```python
from build123d import *

# Parameters (mm, degrees)
BOSS_EXTRUDE1_DEPTH = 152.146
SKETCH2_W           = 2.509536254
SKETCH2_H           = 5.091968042
SKETCH2_W_2         = 2.457399938
BOSS_EXTRUDE2_DEPTH = 2.032
SKETCH3_W           = 5.037993656
SKETCH3_H           = 2.032
BOSS_EXTRUDE3_DEPTH = 2.54
SKETCH4_W           = 5.091968042
SKETCH4_H           = 2.032
BOSS_EXTRUDE4_DEPTH = 2.54


with BuildPart() as part:
    # Sketch1 → Boss-Extrude1 (new body)
    with BuildSketch(Plane(origin=(0, 0, 0), x_dir=(0, 0, -1), z_dir=(1, 0, 0))):
        with BuildLine():
            Line((0, 42.142112298), (36.917745163, 42.142112298))
            ThreePointArc((36.917745163, 42.142112298), (40.509847611, 40.654214746), (41.997745163, 37.062112298))
            Line((41.997745163, 37.062112298), (41.997745163, -12.467887702))
            ThreePointArc((41.997745163, -12.467887702), (40.509847611, -16.05999015), (36.917745163, -17.547887702))
            Line((36.917745163, -17.547887702), (0, -17.547887702))
            Line((0, -17.547887702), (0, -15.515887702))
            Line((0, -15.515887702), (34.644615501, -15.515887702))
            ThreePointArc((34.644615501, -15.515887702), (38.23671795, -14.02799015), (39.724615501, -10.435887702))
            Line((39.724615501, -10.435887702), (39.724615501, 35.036686341))
            ThreePointArc((39.724615501, 35.036686341), (38.23671795, 38.628788789), (34.644615501, 40.116686341))
            Line((34.644615501, 40.116686341), (0, 40.116686341))
            Line((0, 40.116686341), (0, 42.142112298))
        make_face()
    extrude(amount=-BOSS_EXTRUDE1_DEPTH)

    # Sketch2 → Boss-Extrude2 (add)
    with BuildSketch(Plane(origin=(0, 42.142112298, 0), x_dir=(1, 0, 0), z_dir=(0, 1, 0))):
        with Locations((-153.400768127, 10.723169707)):
            Rectangle(SKETCH2_W, SKETCH2_H)
        with Locations((1.228699969, 10.723169707)):
            Rectangle(SKETCH2_W_2, SKETCH2_H)
    extrude(amount=-BOSS_EXTRUDE2_DEPTH)

    # Sketch3 → Boss-Extrude3 (add)
    with BuildSketch(Plane(origin=(0, 0, 0), x_dir=(0, 0, -1), z_dir=(1, 0, 0))):
        with Locations((10.77174546, -16.531887702)):
            Rectangle(SKETCH3_W, SKETCH3_H)
    extrude(amount=BOSS_EXTRUDE3_DEPTH)

    # Sketch4 → Boss-Extrude4 (add)
    with BuildSketch(Plane.ZY.offset(152.146)):
        with Locations((-10.723169707, -16.531887702)):
            Rectangle(SKETCH4_W, SKETCH4_H)
    extrude(amount=BOSS_EXTRUDE4_DEPTH)


solid = part.part
```
Model file for the job. Use its own axes, mm. A direction names the side the tool comes from. Round coordinates to 2 decimals unless told otherwise and drop trailing zeros. Order: outer loops, then holes, each group sorted by start corner. A loop starts at its lowest first (then second) coordinate and runs counter-clockwise, first axis right, second up. Notation, with made-up numbers: (72, -13) -> (96, -13) arc R17 cw to (96, -6) -> close; hole circle Ø6 at (-36, 16.5). An arc over 180 degrees is marked (long way). Use one line per item in the form item = value.
Item 1: Drill centre lines: line 1 (Y direction, x = -20.5, z = -20); line 2 (Z direction, x = -45.5, y = 22); line 3 (Y direction, x = -130, z = -35.5). Where is each one in solid material? Low to high.
Returned:
line_1 = -17.55 to -15.52, 40.12 to 42.14
line_2 = -42 to -39.72
line_3 = -17.55 to -15.44, 40.04 to 42.14
Item 2: Cut at D-D, the plane z = -23.5. Write the cut outline in (x, y).
Returned:
outline = (-152.15, -17.55) -> (0, -17.55) -> (0, -15.52) -> (-152.15, -15.52) -> close; (-152.15, 40.12) -> (0, 40.12) -> (0, 42.14) -> (-152.15, 42.14) -> close
Item 3: Cut at C-C, the plane y = 29.5. Write the cut outline in (x, z), and give its area (3 significant figures).
Returned:
outline = (-152.15, -42) -> (0, -42) -> (0, -39.72) -> (-152.15, -39.72) -> close
area = 346 mm^2
Item 4: Cut at B-B, the plane x = -70. Write the cut outline in (y, z).
Returned:
outline = (-17.55, -36.92) arc R5.08 ccw to (-12.47, -42) -> (37.06, -42) arc R5.08 ccw to (42.14, -36.92) -> (42.14, 0) -> (40.12, 0) -> (40.12, -34.64) arc R5.08 cw to (35.04, -39.72) -> (-10.44, -39.72) arc R5.08 cw to (-15.52, -34.64) -> (-15.52, 0) -> (-17.55, 0) -> close
Item 5: Flat gauge pins, fed straight in: pin 1 Ø1.6 at (x, y) = (-153, -16.5) entering from -Z; pin 2 Ø1 at (x, y) = (-119.5, 2.5) entering from +Z; pin 3 Ø2 at (y, z) = (-16.5, -4) entering from +X. Where does each tip first touch, or does it go through?
Returned:
pin_1 = -13.27
pin_2 = -39.72
pin_3 = 0
Item 6: Tool access for faces 5 (the face through (-75, -15.516, -17)), 6 (the face through (-75, -17.548, -19)), 7 (the face through (0, 15, -40)): list every direction of +Z, -Z, +X, -X, +Y, -Y with a clear straight run to the whole face (end or side of a thin tool).
Returned:
face_5 = +Z, +X, -X
face_6 = +Z, -Z, +X, -X, -Y
face_7 = -Z, +X, +Y, -Y
Item 7: Pull direction Y, two halves, no side cores. Call faces 1 (the face through (-75.008, -14.067, -38.197)), 2 (the face through (-75.008, 40.693, -40.47)), 3 (the face through (-75.01, -16.02, -40.55)), 4 (the face through (-152.146, 15, -40)): released by +Y, released by -Y, zero draft, split by the parting line, or undercut.
Returned:
face_1 = undercut
face_2 = released by +Y
face_3 = released by -Y
face_4 = zero draft
